```python
from build123d import *

# Parameters (mm, degrees)
SKETCH1_W           = 4.5
SKETCH1_H           = 5
BOSS_EXTRUDE1_DEPTH = 1
SKETCH2_R           = 2.25
BOSS_EXTRUDE2_DEPTH = 2.5
BOSS_EXTRUDE3_DEPTH = 0.5
CUT_EXTRUDE1_DEPTH  = 0.05


with BuildPart() as part:
    # Sketch1 → Boss-Extrude1 (new body)
    with BuildSketch(Plane.XY):
        with Locations((-2.25, 2.5)):
            Rectangle(SKETCH1_W, SKETCH1_H)
    extrude(amount=BOSS_EXTRUDE1_DEPTH)

    # Sketch2 → Boss-Extrude2 (add)
    with BuildSketch(Plane.XY.offset(1)):
        with Locations((-2.25, 2.5)):
            Circle(SKETCH2_R)
    extrude(amount=BOSS_EXTRUDE2_DEPTH)

    # Sketch3 → Boss-Extrude3 (add)
    with BuildSketch(Plane.XY.offset(3.5)):
        Polygon((-1.214319799, 5.000353186), (-3.285680201, 5.000353186), (-4.750353186, 3.535680201), (-4.750353186, 1.464319799), (-3.285680201, -0.000353186), (-1.214319799, -0.000353186), (0.250353186, 1.464319799), (0.250353186, 3.535680201), align=None)
    extrude(amount=BOSS_EXTRUDE3_DEPTH)

    # Sketch5 → Cut-Extrude1 (cut)
    with BuildSketch(Plane(origin=(0, 0, 0), x_dir=(-1, 0, 0), z_dir=(0, 0, -1))):
        Polygon((0.25, 5), (0, 5), (0, 0), (0.25, 0), (0.25, 1.25), (4.25, 1.25), (4.25, 0), (4.5, 0), (4.5, 5), (4.25, 5), (4.25, 3.75), (0.25, 3.75), align=None)
    extrude(amount=-CUT_EXTRUDE1_DEPTH, mode=Mode.SUBTRACT)


solid = part.part
```
Could you check a few things on this model? Use its own coordinates, in mm. A direction names the side the tool comes from. Give positions to 0.01 mm unless a question says otherwise; leave off trailing zeros. Order: outer loops, then holes, each group sorted by start corner. A loop starts at its lowest first (then second) coordinate and runs counter-clockwise, first axis right, second up.
Q1. If I drill on line 1 along Z through (x, y) = (-4.3, 1.45); line 2 along Z through (x, y) = (-3.4, 1.45); line 3 along X through (y, z) = (1.05, 0.95), over which ranges is the centre line in solid material (lowest first)?
Q2. For faces 1 (the flat face through (-0.492, 0.722, 3.746)), 2 (the flat face through (-0.472, 4.258, 3.746)), 3 (the flat face through (-4.028, 0.742, 3.746)), 4 (the flat face through (-4.5, 2.5, 0.5)), 5 (the flat face through (0, 2.5, 0.5)), which set-ups out of +Z, -Z, +X, -X, +Y, -Y let a thin tool reach every point of the face, with its end or its side?
Q3. Suppose I cut it at D-D, the plane x = -0.9. Write out the boundary of the cut face in (y, z), and give its area (3 significant figures).
Q4. Suppose I cut it at C-C, the plane z = 1.95. Write out the boundary of the cut face in (x, y), and give its area (3 significant figures).
Q5. We'd pull the mould along Z, two halves only. Please class faces 6 (the cylindrical face through (-2.738, 0.304, 2.232)), 7 (the flat face through (-2, 3, 4)), 8 (the flat face through (-4.008, 4.278, 3.746)): +Z half, -Z half, draft (parallel to the pull), parting line (faces both ways), or undercut.
Q6. I'm going to push flat-ended pins straight in: P1, Ø0.5, axis at y = 1.5, z = 0.5, coming from the +X side; P2, Ø2, axis at x = -3, y = 1.5, coming from the -Z side. Where does each tip first touch, or does it pass through?
Q7. Suppose I cut it at A-A, the plane x = -2.25. Write out the boundary of the cut face in (y, z), and give its area (3 significant figures).
Solution:
1. line 1: z = 0.05 to 1, 3.5 to 4
1. line 2: z = 0.05 to 4
1. line 3: x = -4.5 to 0
2. face 1: +Z, +X, -Y
2. face 2: +Z, +X, +Y
2. face 3: +Z, -X, -Y
2. face 4: -Z, -X, +Y, -Y
2. face 5: -Z, +X, +Y, -Y
3. outline: (0, 0) - (1.25, 0) - (1.25, 0.05) - (3.75, 0.05) - (3.75, 0) - (5, 0) - (5, 1) - (4.3, 1) - (4.3, 3.5) - (4.69, 3.5) - (4.69, 4) - (0.31, 4) - (0.31, 3.5) - (0.7, 3.5) - (0.7, 1) - (0, 1) - close
3. area: 16.1 mm2
4. outline: circle Ø4.5 at (-2.25, 2.5)
4. area: 15.9 mm2
5. face 6: undercut
5. face 7: +Z half
5. face 8: draft
6. P1: stops at x = 0
6. P2: stops at z = 0
7. outline: (0, 0) - (1.25, 0) - (1.25, 0.05) - (3.75, 0.05) - (3.75, 0) - (5, 0) - (5, 1) - (4.75, 1) - (4.75, 3.5) - (5, 3.5) - (5, 4) - (0, 4) - (0, 3.5) - (0.25, 3.5) - (0.25, 1) - (0, 1) - close
7. area: 18.6 mm2
